For this review, use the dimensioned drawing (mm, ordinates from the lowest corner) and the shaded views. A direction names the side the tool comes from. Round coordinates to 2 decimals unless told otherwise and drop trailing zeros. Write each loop counter-clockwise with the first axis right and the second up, starting at its lowest first coordinate (ties: lowest second). Pieces come first, ordered by that corner, then holes. Notation, with made-up numbers: M 44,-22.75 L 60,-22.75 A26 cw 60,9.25 Z; hole C 89.25,-29 d2. An arc over 180 degrees is marked long. One line per question, with ' | ' between items. Start each with the question number.
Item 1: Add section D-D, the plane y = 3. State the section outline as (x, z) points.
Item 2: Draft analysis for pull direction X (two halves, no side actions). For the marked faces 1, 2, 3 and 4, state which applies: released by +X, released by -X, zero draft, split by the parting line, or undercut.
Item 3: Add section B-B, the plane z = 96. State the section outline as (x, y) points, and give its area (3 significant figures).
Item 4: Machinability: for the marked faces 5, 6 and 7, which of the approach directions +Z, -Z, +X, -X, +Y, -Y give a long, thin tool a straight path to every point of the face, cutting with its end or side? Answer none if there is none.
Item 5: For L1, parallel to X at y = 32.5, z = 131; L2, parallel to Y at x = 61, z = 86; L3, parallel to X at y = 27.5, z = 35, list the stretches that pass through material, from the lowest coordinate up.
Item 6: Insertion check: pin 1 Ø8 at (x, y) = (96, 23) entering from -Z; pin 2 Ø12 at (y, z) = (28, 18) entering from +X; pin 3 Ø12 at (y, z) = (31, 131) entering from -X; pin 4 Ø10 at (x, y) = (29.5, 8.5) entering from +Z. Each pin has a flat end and moves straight along its axis. Give the tip position at first contact, or say it passes through.
Item 7: Add section C-C, the plane x = 77. State the section outline as (y, z) points, and give its area (3 significant figures).
Item 8: Add section A-A, the plane y = 13. State the section outline as (x, z) points.
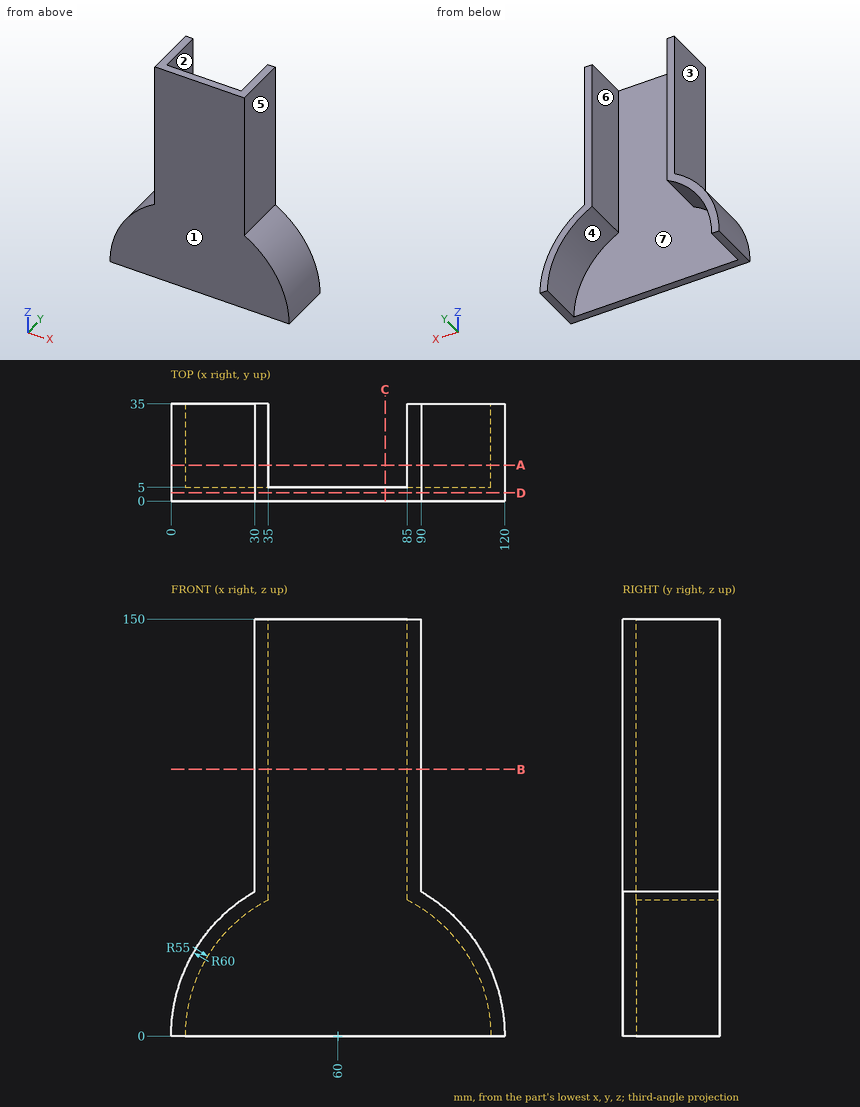
Computed values:
1) outline: M 0,0 L 120,0 A60 ccw 90,51.96 L 90,150 L 30,150 L 30,51.96 A60 ccw Z
2) face 1: zero draft | face 2: undercut | face 3: released by -X | face 4: undercut
3) outline: M 30,0 L 90,0 L 90,35 L 85,35 L 85,5 L 35,5 L 35,35 L 30,35 Z | area: 600 mm^2
4) face 5: +Z, +X, +Y, -Y | face 6: +Z, -Z, +Y | face 7: -Z, +Y
5) L1: x = 30 to 35, 85 to 90 | L2: y = 0 to 5 | L3: x = 11.27 to 17.57, 102.43 to 108.73
6) pin 1: stops at z = 37.75 | pin 2: stops at x = 118.79 | pin 3: stops at x = 30 | pin 4: stops at z = 150
7) outline: M 0,0 L 5,0 L 5,150 L 0,150 Z | area: 750 mm^2
8) outline: M 0,0 L 5,0 A55 cw 35,48.99 L 35,150 L 30,150 L 30,51.96 A60 ccw Z; M 85,48.99 A55 cw 115,0 L 120,0 A60 ccw 90,51.96 L 90,150 L 85,150 Z
